Autodesk Inventor part; units mm, degrees
ref_plane "YZ Plane" through (0, 0, 0) normal (1, 0, 0) x (0, 1, 0)
ref_plane "XZ Plane" through (0, 0, 0) normal (0, 1, 0) x (-1, 0, 0)
ref_plane "XY Plane" through (0, 0, 0) normal (0, 0, 1) x (1, 0, 0)
sketch "スケッチ1" plane through (0, 0, 0) normal (0, 0, 1) x (1, 0, 0)
  line L0 (0, 0) -> (20, 0)
  line L1 (20, 0) -> (20, 50)
  line L2 (20, 50) -> (0, 50)
  line L3 (0, 50) -> (0, 0)
  dimension "d0" = 20
  dimension "d1" = 50
extrude "押し出し1" add sketch "スケッチ1" along normal blind 10
sketch "スケッチ2" plane through (0, 0, 10) normal (0, 0, 1) x (1, 0, 0)
  line L0 (20, 50) -> (0, 50)
  line L1 (4, 50) -> (16, 50)
  line L2 (16, 50) -> (16, 40)
  line L3 (16, 40) -> (4, 40)
  line L4 (4, 40) -> (4, 50)
  line L5 (0, 50) -> (0, 0)
  dimension "d4" = 12
  dimension "d5" = 4
  dimension "d6" = 10
extrude "押し出し2" cut sketch "スケッチ2" against normal blind 10
sketch "スケッチ3" plane through (20, 0, 0) normal (1, 0, 0) x (0, 0, -1)
  line L0 (0, 50) -> (-10, 50)
  line L1 (0, 0) -> (0, 50)
  point P0 (-5, 45)
  dimension "d9" = 5
  dimension "d10" = 5
hole "穴1" at (20, 45, 5) direction (-1, 0, 0) diameter 6 end through all
sketch "スケッチ4" plane through (0, 0, 0) normal (0, -1, 0) x (1, 0, 0)
  line L0 (0, 0) -> (0, 10)
  line L1 (0, 10) -> (20, 10)
  line L2 (0, 0) -> (20, 0)
  line L3 (20, 0) -> (20, 10)
  point P0 (5, 5)
  point P1 (15, 5)
  dimension "d18" = 5
  dimension "d19" = 5
  dimension "d20" = 5
  dimension "d21" = 5
hole "穴2" at (5, 0, 5) at (15, 0, 5) direction (0, 1, 0) diameter 2.459 depth 25 tip angle 118
sketch "スケッチ5" plane through (0, 0, 10) normal (0, 0, 1) x (1, 0, 0)
  line L0 (4, 40) -> (16, 40)
  line L1 (4, 40) -> (16, 40)
  line L2 (16, 40) -> (16, 35)
  line L3 (16, 35) -> (4, 35)
  line L4 (4, 35) -> (4, 40)
  point P0 (0, 0)
  dimension "d29" = 5
extrude "押し出し3" cut sketch "スケッチ5" against normal blind 10
sketch "スケッチ6" plane through (0, 0, 10) normal (0, 0, 1) x (1, 0, 0)
  line L0 (0, 50) -> (0, 0)
  line L1 (20, 0) -> (20, 50)
  line L2 (0, 5) -> (20, 5)
  line L3 (20, 5) -> (20, 0)
  line L4 (20, 0) -> (0, 0)
  line L5 (0, 0) -> (0, 5)
  point P0 (20, 5)
  dimension "d32" = 5
extrude "押し出し4" cut sketch "スケッチ6" against normal blind 10
properties part number "アーム支え"
Input: part model. Units: mm. Frame: model coordinates. A direction names the side the tool comes from. Coordinates: 2 decimals unless noted, no trailing zeros. Write each loop counter-clockwise with the first axis right and the second up, starting at its lowest first coordinate (ties: lowest second). Pieces come first, ordered by that corner, then holes. Notation, with made-up numbers: (60.5, 39) - (68.5, 39) arc R14 cw to (68.5, 43) - close; hole circle Ø11 at (-31, 39.25). An arc over 180 degrees is marked (long way). Put each result on its own line as item: value. Start each with the question number.
1) Cut plane D-D (z = 2.75). Return the cut outline in (x, y).
2) Mould query, pull axis X, two halves, no side actions, for faces 4 (the face through (20, 27, 5)), 5 (the face through (2, 42, 5)), 6 (the face through (4, 41, 5)), 7 (the face through (0, 28, 5)). Classes: pulls with the +X half, pulls with the -X half, needs draft (parallel to the pull), parting line crosses it, or undercut.
3) Ray query, L1, parallel to Y at x = 0.8, z = 5; L2, parallel to Z at x = 18.55, y = 45; L3, parallel to X at y = 37, z = 2.25. Return the intervals inside material, ascending.
4) Cut plane A-A (y = 45). Return the cut outline in (x, z), plus the area to 3 significant figures.
5) Cut plane B-B (z = 8.75). Return the cut outline in (x, y), plus the area to 3 significant figures.
6) Reachability of faces 1 (the face through (10, 35, 5)), 2 (the face through (13.78, 15.14, 5.16)), 3 (the face through (10, 23, 0)) from +Z, -Z, +X, -X, +Y, -Y: full face, straight path, thin tool, end or side. Return the list, or none.
7) Contact query for flat-ended pins moving along their axis: pin 1 (1.5 mm diameter, centred on x = 5, z = 5, fed in from +Y); pin 2 (3.5 mm diameter, centred on y = 45, z = 5, fed in from -X). Output: stop coordinate, or through.
8) Cut plane C-C (x = 17.25). Return the cut outline in (y, z), plus the area to 3 significant figures.
Resolved:
1. outline: (0, 5) - (20, 5) - (20, 43.02) - (16, 43.02) - (16, 35) - (4, 35) - (4, 43.02) - (0, 43.02) - close; (0, 46.98) - (4, 46.98) - (4, 50) - (0, 50) - close; (16, 46.98) - (20, 46.98) - (20, 50) - (16, 50) - close
2. face 4: pulls with the +X half
2. face 5: needs draft
2. face 6: undercut
2. face 7: pulls with the -X half
3. L1: y = 5 to 42, 48 to 50
3. L2: z = 0 to 2, 8 to 10
3. L3: x = 0 to 4, 16 to 20
4. outline: (0, 0) - (4, 0) - (4, 2) - (0, 2) - close; (0, 8) - (4, 8) - (4, 10) - (0, 10) - close; (16, 0) - (20, 0) - (20, 2) - (16, 2) - close; (16, 8) - (20, 8) - (20, 10) - (16, 10) - close
4. area: 32.0 mm2
5. outline: (0, 5) - (20, 5) - (20, 50) - (16, 50) - (16, 35) - (4, 35) - (4, 50) - (0, 50) - close
5. area: 720 mm2
6. face 1: +Z, -Z, +Y
6. face 2: -Y
6. face 3: -Z, +X, -X, +Y, -Y
7. pin 1: stops at y = 35
7. pin 2: passes through
8. outline: (5, 0) - (50, 0) - (50, 10) - (5, 10) - close; hole circle Ø6 at (45, 5)
8. area: 422 mm2
